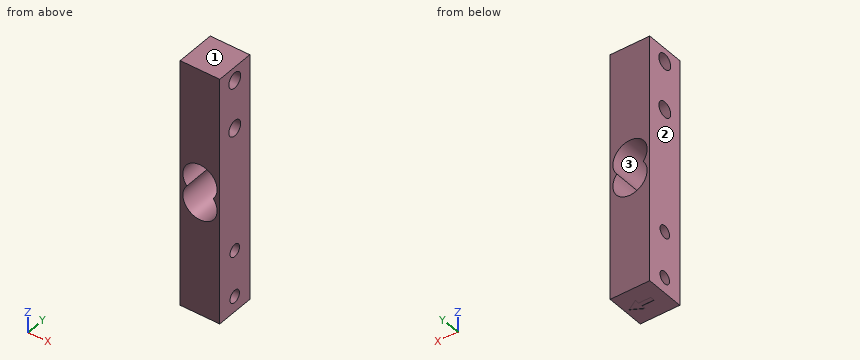
Autodesk Inventor part; units mm, degrees
ref_plane "YZ Plane" through (0, 0, 0) normal (1, 0, 0) x (0, 1, 0)
ref_plane "XZ Plane" through (0, 0, 0) normal (0, 1, 0) x (-1, 0, 0)
ref_plane "XY Plane" through (0, 0, 0) normal (0, 0, 1) x (1, 0, 0)
sketch "Sketch1" plane through (0, 0, 0) normal (0, 1, 0) x (-1, 0, 0)
  line L0 (0, 0) -> (12.7, 0)
  line L1 (12.7, 0) -> (12.7, -80)
  line L2 (12.7, -80) -> (0, -80)
  line L3 (0, -80) -> (0, 0)
  circle A0 centre (6.35, -36.5) radius 5.5
  circle A1 centre (6.35, -43.5) radius 5.5
  line L4 (6.35, -36.5) -> (6.35, -43.5) construction
  point P0 (6.35, -40)
  point P1 (0, -40)
  point P2 (6.35, -80)
  dimension "d0" = 12.7
  dimension "d1" = 80
  dimension "d2" = 11
  dimension "d3" = 11
  dimension "d4" = 7
extrude "Extrusion1" add sketch "Sketch1" along normal blind 12.7
sketch "Sketch2" plane through (-12.7, 0, -80) normal (-1, 0, 0) x (0, 0, 1)
  line L0 (40, 0) -> (40, 12.7)
  line L1 (40, 6.35) -> (20, 6.35) construction
  line L2 (20, 6.35) -> (5, 6.35) construction
  circle A0 centre (5, 6.35) radius 2
  circle A1 centre (20, 6.35) radius 2
  line L3 (40, 6.35) -> (60, 6.35) construction
  line L4 (60, 6.35) -> (75, 6.35) construction
  circle A2 centre (60, 6.35) radius 2.5
  circle A3 centre (75.6534, 6.35) radius 2.5
  point P0 (80, 0)
  dimension "d7" = 20
  dimension "d8" = 15
  dimension "d9" = 4
  dimension "d10" = 4
  dimension "d11" = 5
  dimension "d12" = 5
sketch "Sketch3" plane through (0, 0, -80) normal (0, 0, -1) x (-1, 0, 0)
  line L0 (8.7436, 7.084) -> (3.6466, 7.084)
  line L1 (3.6466, 7.084) -> (3.6466, 5.616)
  line L2 (3.6466, 5.616) -> (8.7436, 5.616)
  line L3 (8.7436, 5.616) -> (8.7436, 7.084)
  line L4 (8.7436, 7.084) -> (3.6466, 5.616) construction
  line L5 (3.6466, 7.084) -> (8.7436, 5.616) construction
  line L6 (1.2106, 6.35) -> (4.8647, 8.4597)
  line L7 (4.8647, 8.4597) -> (4.8647, 4.2403)
  line L8 (4.8647, 4.2403) -> (1.2106, 6.35)
  point P0 (0, 0)
  point P1 (6.1951, 6.35)
  point P2 (3.6466, 6.35)
extrude "Extrusion2" cut sketch "Sketch3" against normal blind 0.1
extrude "Extrusion3" cut sketch "Sketch2" against normal through all
properties part number "LoadCell"
Geometry check sheet. Reference: the model listing, model coordinates, mm. Face numbers are marked on the shaded views. Coordinates: 2 decimals unless noted, no trailing zeros. Order: outer loops, then holes, each group sorted by start corner. A loop starts at its lowest first (then second) coordinate and runs counter-clockwise, first axis right, second up. Notation, with made-up numbers: M 30.5,61 L 37.5,61 A18 cw 37.5,91 Z; hole C 0,8 d9. An arc over 180 degrees is marked long. Use CSV: the item, a comma, the result in double quotes.
Item 1: Gauge pin test, flat ends, axial feed: pin 1 Ø5 at (y, z) = (6.35, -75) entering from -X; pin 2 Ø4 at (y, z) = (6.35, -4.35) entering from -X. Record the tip position at first contact, or that the pin passes through.
Returned:
pin 1,"stops at x = -12.7"
pin 2,"passes through"
Item 2: Cross-section at D-D on y = 11.25. Record the cut outline in (x, z), then the cut area to 3 significant figures.
Returned:
outline,"M -12.7,-80 L 0,-80 L 0,0 L -12.7,0 Z; hole M -10.59,-40 A5.5 ccw long -2.11,-40 A5.5 ccw long Z"
area,"850 mm2"
Item 3: Mould release check, pull along X, two halves, no side actions. Record for the marked faces 1, 2 and 3: pulls with the +X half, pulls with the -X half, needs draft (parallel to the pull), parting line crosses it, or undercut.
Returned:
face 1,"needs draft"
face 2,"pulls with the -X half"
face 3,"undercut"
Item 4: Cross-section at B-B on z = -75. Record the cut outline in (x, y).
Returned:
outline,"M -12.7,0 L 0,0 L 0,4.35 L -12.7,4.35 Z; M -12.7,8.35 L 0,8.35 L 0,12.7 L -12.7,12.7 Z"
Item 5: Cross-section at A-A on x = -6.35. Record the cut outline in (y, z).
Returned:
outline,"M 0,-80 L 5.62,-80 L 5.62,-79.9 L 7.08,-79.9 L 7.08,-80 L 12.7,-80 L 12.7,-49 L 0,-49 Z; M 0,-31 L 12.7,-31 L 12.7,0 L 0,0 Z; hole C 6.35,-20 d5; hole C 6.35,-4.35 d5; hole C 6.35,-75 d4; hole C 6.35,-60 d4"
Item 6: Thickness scan on line 1 along Y through (x, z) = (-3.5, -75); line 2 along Z through (x, y) = (-6.25, 9); line 3 along X through (y, z) = (8.25, -36.5). Record the ranges inside material, lowest first.
Returned:
line 1,"y = 0 to 4.35, 8.35 to 12.7"
line 2,"z = -80 to -49, -31 to 0"
line 3,"x = -12.7 to -11.85, -0.85 to 0"
Item 7: Cross-section at C-C on z = -20. Record the cut outline in (x, y), then the cut area to 3 significant figures.
Returned:
outline,"M -12.7,0 L 0,0 L 0,3.85 L -12.7,3.85 Z; M -12.7,8.85 L 0,8.85 L 0,12.7 L -12.7,12.7 Z"
area,"97.8 mm2"
